Check sheet for the modelled part. Datum: model origin and axes. Units: mm. Face numbers are marked on the shaded views. Round coordinates to 2 decimals unless told otherwise and drop trailing zeros. Write each loop counter-clockwise with the first axis right and the second up, starting at its lowest first coordinate (ties: lowest second). Pieces come first, ordered by that corner, then holes. Notation, with made-up numbers: (22, 41) - (47, 41) arc R14 ccw to (47, 64) - close; hole circle Ø1 at (51, 73). An arc over 180 degrees is marked (long way). Answer as a JSON object with one key per item and string values. Group by question number.
Item 1: Thickness scan on line 1 (Z direction, x = -13, y = 0); line 2 (Y direction, x = -6, z = 15) (3 decimals); line 3 (Y direction, x = -19, z = 1) (3 decimals). Record the ranges inside material, lowest first.
Item 2: Sectioned sample at B-B on z = 0. Record the boundary of the cut face in (x, y) (1 decimal), plus the area to 3 significant figures.
Item 3: Gauge pin test, flat ends, axial feed: P1, Ø4, axis at y = 1, z = 10, coming from the -X side; P2, Ø1, axis at x = -19.5, y = -2, coming from the -Z side. Record the tip position at first contact, or that the pin passes through.
Item 4: Sectioned sample at A-A on y = 0. Record the boundary of the cut face in (x, z), plus the area to 3 significant figures.
Item 5: Sectioned sample at D-D on z = 11.75. Record the boundary of the cut face in (x, y) (3 decimals).
Item 6: Release check for a two-part mould opening along Z. For the marked faces 1 and 2 record: pulls with the +Z half, pulls with the -Z half, needs draft (parallel to the pull), parting line crosses it, or undercut.
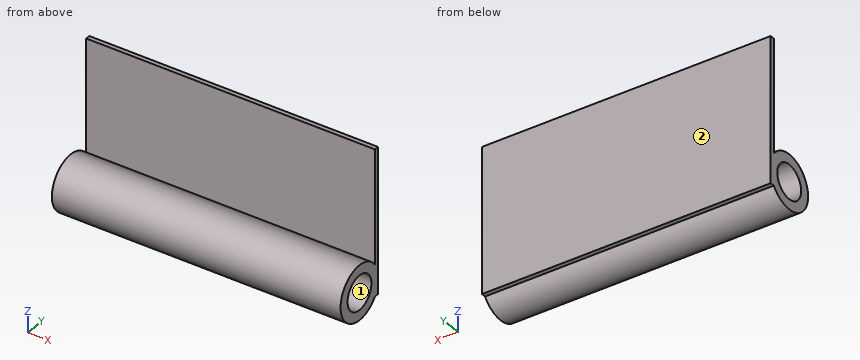
Autodesk Inventor part; units mm, degrees
ref_plane "YZ Plane" through (0, 0, 0) normal (1, 0, 0) x (0, 1, 0)
ref_plane "XZ Plane" through (0, 0, 0) normal (0, 1, 0) x (-1, 0, 0)
ref_plane "XY Plane" through (0, 0, 0) normal (0, 0, 1) x (1, 0, 0)
sketch "Sketch1" plane through (0, 0, 0) normal (1, 0, 0) x (0, 1, 0)
  circle A0 centre (0, 0) radius 3
  circle A1 centre (0, 0) radius 4.7625
  line L0 (4.7625, 0) -> (3, 0)
  line L1 (3.8813, 0) -> (3.8813, 2.7599)
  line L2 (3.8813, 0) -> (3.8813, -2.7599)
  dimension "d0" = 6
extrude "Extrusion1" add sketch "Sketch1" against normal blind 50.8 contours L2 A1 L1
sketch "Sketch2" plane through (0, 3.8813, 2.7599) normal (0, 1, 0) x (1, 0, 0)
  line L0 (0, 5.5199) -> (-50.8, 5.5199)
  line L1 (0, 5.5199) -> (-50.8, 5.5199)
  line L2 (-50.8, 5.5199) -> (-50.8, -19.8801)
  line L3 (-50.8, -19.8801) -> (0, -19.8801)
  line L4 (0, -19.8801) -> (0, 5.5199)
  point P0 (0, 0)
  dimension "d7" = 50.8
  dimension "d8" = 25.4
extrude "Extrusion2" add sketch "Sketch2" along normal blind 0.7937
properties part number "AxleHolder_3DPrint"
Completed:
{
 "1": {"line 1": "-4.76 to -3, 3 to 4.76", "line 2": "3.881 to 4.675", "line 3": "-4.656 to -2.828, 2.828 to 4.675"},
 "2": {"outline": "(-50.8, -4.8) - (0, -4.8) - (0, -3) - (-50.8, -3) - close; (-50.8, 3) - (0, 3) - (0, 4.7) - (-50.8, 4.7) - close", "area": "175 mm²"},
 "3": {"P1": "through", "P2": "z = -4.52"},
 "4": {"outline": "(-50.8, -4.76) - (0, -4.76) - (0, -3) - (-50.8, -3) - close; (-50.8, 3) - (0, 3) - (0, 4.76) - (-50.8, 4.76) - close", "area": "179 mm²"},
 "5": {"outline": "(-50.8, 3.881) - (0, 3.881) - (0, 4.675) - (-50.8, 4.675) - close"},
 "6": {"face 1": "undercut", "face 2": "needs draft"}
}
